Autodesk Inventor part; units mm, degrees
ref_plane "YZ Plane" through (0, 0, 0) normal (1, 0, 0) x (0, 1, 0)
ref_plane "XZ Plane" through (0, 0, 0) normal (0, 1, 0) x (-1, 0, 0)
ref_plane "XY Plane" through (0, 0, 0) normal (0, 0, 1) x (1, 0, 0)
sketch "Sketch1" plane through (0, 0, 0) normal (0, 0, 1) x (1, 0, 0)
  line L0 (0, 0) -> (104, 0)
  line L1 (104, 0) -> (104, 54.5)
  line L2 (104, 54.5) -> (0, 54.5)
  line L3 (0, 54.5) -> (0, 10)
  circle A0 centre (96, 27.25) radius 1.625
  circle A1 centre (17, 41.25) radius 1.625
  circle A2 centre (17, 13.25) radius 1.625
  line L4 (0, 0) -> (-10, 0)
  line L5 (-10, 0) -> (-10, 10)
  line L6 (-10, 10) -> (0, 10)
  dimension "d0" = 104
  dimension "d1" = 54.5
  dimension "d9" = 28
  dimension "d10" = 13.25
  dimension "d11" = 17
  dimension "d12" = 3.25
  dimension "d13" = 3.25
  dimension "d14" = 17
  dimension "d15" = 8
  dimension "d16" = 3.25
  dimension "d17" = 27.25
  dimension "d34" = 10
  dimension "d35" = 10
extrude "Main Mount" add sketch "Sketch1" along normal blind 3
sketch "Sketch2" plane through (0, 0, 0) normal (0, -1, 0) x (1, 0, 0)
  line L0 (104, 0) -> (0, 0)
  line L1 (0, 0) -> (104, 0)
  line L2 (0, 0) -> (-55, 0)
  line L3 (-55, 0) -> (-55, 43)
  line L4 (-55, 43) -> (104, 43)
  line L5 (104, 43) -> (104, 0)
  line L6 (104, 0) -> (0, 0)
  dimension "d20" = 55
  dimension "d21" = 43
extrude "Base" add sketch "Sketch2" along normal blind 3
sketch "Sketch3" plane through (0, 0, 0) normal (0, 1, 0) x (1, 0, 0)
  line L0 (-55, 0) -> (-52, 0)
  line L1 (-55, 0) -> (104, 0)
  line L2 (-52, -43) -> (-55, -43)
  line L3 (-55, -43) -> (-55, 0)
  line L4 (-55, -43) -> (-55, 0)
  line L5 (-52, -17.5) -> (-55, -17.5)
  line L6 (-55, -43) -> (-55, 0)
  line L7 (-52, -25.5) -> (-55, -25.5)
  line L8 (-52, 0) -> (-52, -17.5)
  line L9 (-52, -25.5) -> (-52, -43)
  dimension "d24" = 3
  dimension "d31" = 8
extrude "Laser Mount" add sketch "Sketch3" along normal blind 55
hole "Cable Management" at (-5, 5, 3) direction (0, 0, -1) diameter 6.5 depth 8 tip angle 118
hole "Cable Routing" at (-52, 5, 5) direction (-1, 0, 0) diameter 4 depth 8 tip angle 118
fillet "Strength" radius 4 10 edges at (-52, 0, 8.75) (-52, 0, 34.25) (-53.5, 55, 43) (-53.5, 55, 0) (47, 0, 3) (-10, 0, 1.5) (-10, 10, 1.5) (0, 10, 1.5) (0, 54.5, 1.5) (104, 54.5, 1.5)
properties part number "LaserMount"
For this review, take the finished solid that the model builds, in its own axes (mm). A direction names the side the tool comes from. Round coordinates to 2 decimals unless told otherwise and drop trailing zeros. Order: outer loops, then holes, each group sorted by start corner. A loop starts at its lowest first (then second) coordinate and runs counter-clockwise, first axis right, second up. Notation, with made-up numbers: (-20, 80) -> (-6, 80) arc R35 cw to (-6, 113) -> close; hole circle Ø2 at (-16, 83.5). An arc over 180 degrees is marked (long way). Write item = value, one per line. Start each with the question number.
1) Insertion check: pin 1 (1.5 mm diameter, centred on x = 7, y = 48, fed in from +Z); pin 2 (3.5 mm diameter, centred on x = 66, z = 1, fed in from +Y); pin 3 (6 mm diameter, centred on y = 7, z = 18, fed in from +X); pin 4 (3 mm diameter, centred on y = 5, z = 5, fed in from +X). Each pin has a flat end and moves straight along its axis. Give the tip position at first contact, or say it passes through.
2) The part is to be moulded in two halves that separate along Z. For faces 4 (the face through (-52, 29, 34)), 5 (the face through (-53, 27, 25.5)), 6 (the face through (-53.521, 53.859, 1.203)), say which applies: +Z half, -Z half, draft (parallel to the pull), parting line (faces both ways), or undercut.
3) Take a section at C-C on x = 96. State the section outline as (y, z) points (3 decimals), plus the area to 3 significant figures.
4) Take a section at B-B on x = 17. State the section outline as (y, z) points (3 decimals).
5) Tool access review of faces 1 (the face through (45.826, 1.141, 4.203)), 2 (the face through (0, 33, 1)), 3 (the face through (-54, 28, 17.5)): name each direction out of +Z, -Z, +X, -X, +Y, -Y from which nothing blocks a thin tool from reaching the whole face with its end or side.
6) Take a section at D-D on y = 36. State the section outline as (x, z) points.
7) Take a section at A-A on y = 27.25. State the section outline as (x, z) points (3 decimals).
8) To check wall thickness, follow line 1 (X direction, y = 5, z = 1); line 2 (Y direction, x = 17, z = 1.55) (3 decimals); line 3 (X direction, y = 27, z = 1). State the ranges of each line that lie inside material, in increasing order. Write a range as from..to.
Verdict:
q1.pin_1 = 3
q1.pin_2 = 54.5
q1.pin_3 = -52
q1.pin_4 = through
q2.face_4 = draft
q2.face_5 = undercut
q2.face_6 = -Z half
q3.outline = (-3, 0) -> (25.625, 0) -> (25.625, 3) -> (4, 3) arc R4 cw to (0, 7) -> (0, 43) -> (-3, 43) -> close; (28.875, 0) -> (54.5, 0) -> (54.5, 3) -> (28.875, 3) -> close
q3.area = 286 mm2
q4.outline = (-3, 0) -> (11.625, 0) -> (11.625, 3) -> (4, 3) arc R4 cw to (0, 7) -> (0, 43) -> (-3, 43) -> close; (14.875, 0) -> (39.625, 0) -> (39.625, 3) -> (14.875, 3) -> close; (42.875, 0) -> (54.5, 0) -> (54.5, 3) -> (42.875, 3) -> close
q5.face_1 = +Z, +X, +Y
q5.face_2 = +Z, -Z, +Y
q5.face_3 = +X, -X, +Y
q6.outline = (-55, 0) -> (-52, 0) -> (-52, 17.5) -> (-55, 17.5) -> close; (-55, 25.5) -> (-52, 25.5) -> (-52, 43) -> (-55, 43) -> close; (0, 0) -> (104, 0) -> (104, 3) -> (0, 3) -> close
q7.outline = (-55, 0) -> (-52, 0) -> (-52, 17.5) -> (-55, 17.5) -> close; (-55, 25.5) -> (-52, 25.5) -> (-52, 43) -> (-55, 43) -> close; (0, 0) -> (94.375, 0) -> (94.375, 3) -> (0, 3) -> close; (97.625, 0) -> (104, 0) -> (104, 3) -> (97.625, 3) -> close
q8.line_1 = -55..-52, -10..-8.25, -1.75..104
q8.line_2 = -3..11.625, 14.875..39.625, 42.875..54.5
q8.line_3 = -55..-52, 0..94.39, 97.61..104
